Part model, mm, in its own coordinate system. A direction names the side the tool comes from. Give positions to 0.01 mm unless a question says otherwise; leave off trailing zeros. Order: outer loops, then holes, each group sorted by start corner. A loop starts at its lowest first (then second) coordinate and runs counter-clockwise, first axis right, second up. Notation, with made-up numbers: M -22.75,17 L 6.25,17 A36 cw 6.25,52 Z; hole C 52.5,31 d4. An arc over 180 degrees is marked long. Answer as a JSON object with one key per item and string values.
from build123d import *

# Parameters (mm, degrees)
BOSS_EXTRUDE1_DEPTH = 3
FILLET1_R           = 3
SKETCH2_R           = 3
BOSS_EXTRUDE2_DEPTH = 7
SKETCH3_R           = 1.25
CUT_EXTRUDE1_DEPTH  = 11
SKETCH4_R           = 2.125
CUT_EXTRUDE2_DEPTH  = 4


with BuildPart() as part:
    # Sketch1 → Boss-Extrude1 (new body)
    with BuildSketch(Plane(origin=(0, 0, 0), x_dir=(1, 0, 0), z_dir=(0, 1, 0))):
        Polygon((81.303847577, 152.822394855), (113.635462652, 208.822394855), (237.663230149, -6), (173, -6), align=None)
    extrude(amount=BOSS_EXTRUDE1_DEPTH)

    # Fillet1
    fillet1_edges = [part.edges().sort_by_distance(p)[0] for p in [
        (173, 1.5, 6),
        (81.303847577, 1.5, -152.822394855),
        (113.635462652, 1.5, -208.822394855),
        (237.663230149, 1.5, 6),
    ]]
    fillet(fillet1_edges, radius=FILLET1_R)

    # Sketch2 → Boss-Extrude2 (add)
    with BuildSketch(Plane(origin=(0, 3, 0), x_dir=(1, 0, 0), z_dir=(0, 1, 0))):
        with Locations((110.683012702, 108.936188175)):
            Circle(SKETCH2_R)
        with Locations((153.118257487, 133.436188175)):
            Circle(SKETCH2_R)
        with Locations((182.118257487, 83.206714755)):
            Circle(SKETCH2_R)
        with Locations((139.683012702, 58.706714755)):
            Circle(SKETCH2_R)
    extrude(amount=BOSS_EXTRUDE2_DEPTH)

    # Sketch3 → Cut-Extrude1 (cut, through all)
    with BuildSketch(Plane(origin=(0, 10, 0), x_dir=(1, 0, 0), z_dir=(0, 1, 0))):
        with Locations((110.683012702, 108.936188175)):
            Circle(SKETCH3_R)
        with Locations((153.118257487, 133.436188175)):
            Circle(SKETCH3_R)
        with Locations((182.118257487, 83.206714755)):
            Circle(SKETCH3_R)
        with Locations((139.683012702, 58.706714755)):
            Circle(SKETCH3_R)
    extrude(amount=-CUT_EXTRUDE1_DEPTH, mode=Mode.SUBTRACT)

    # Sketch4 → Cut-Extrude2 (cut, through all)
    with BuildSketch(Plane(origin=(0, 3, 0), x_dir=(1, 0, 0), z_dir=(0, 1, 0))):
        with Locations((87.767949192, 152.018547277)):
            Circle(SKETCH4_R)
        with Locations((114.099564267, 197.626242432)):
            Circle(SKETCH4_R)
        with Locations((175.535898385, 0)):
            Circle(SKETCH4_R)
        with Locations((228.199128534, 0)):
            Circle(SKETCH4_R)
    extrude(amount=-CUT_EXTRUDE2_DEPTH, mode=Mode.SUBTRACT)


solid = part.part
1. Which spindle directions (+Z, -Z, +X, -X, +Y, -Y) get a long thin tool onto all of the face, cutting with end or side? Do faces 4 (the flat face through (96.4, 1.48, -178.97)), 5 (the cylindrical face through (154.731, 6.451, -135.966)). Say none if no direction does.
Worked answers:
{"face 4": "-Z, -X, +Y, -Y", "face 5": "+Y"}
2. Pin check, flat tips, straight feed: P1, Ø4, axis at x = 175.54, z = 0, coming from the -Y side; P2, Ø1.5, axis at y = 7, z = -80, coming from the -X side; P3, Ø3, axis at x = 182.12, z = -83.21, coming from the -Y side; P4, Ø4, axis at y = 7.5, z = -135, coming from the +X side. Stop position of each tip, or through.
Worked answers:
{"P1": "passes through", "P2": "stops at x = 180.4", "P3": "stops at y = 0", "P4": "stops at x = 156.12"}
3. Cut at C-C on x = 198.5. Give the cut face in (y, z).
Worked answers:
{"outline": "M 0,-61.83 L 3,-61.83 L 3,6 L 0,6 Z"}
4. Cut at A-A on y = 4.75. Give the cut face in (x, z), plus the area to 3 significant figures.
Worked answers:
{"outline": "C 110.68,-108.94 d6; C 139.68,-58.71 d6; C 153.12,-133.44 d6; C 182.12,-83.21 d6; hole C 110.68,-108.94 d2.5; hole C 139.68,-58.71 d2.5; hole C 153.12,-133.44 d2.5; hole C 182.12,-83.21 d2.5", "area": "93.5 mm^2"}
5. Two-plate mould, pull along X, no slides. Class faces 1 (the cylindrical face through (173.413, 1.521, -0.093)), 2 (the flat face through (153, 10, -132)), 3 (the cylindrical face through (183.503, 6.451, -80.545)): +X half, -X half, draft (parallel to the pull), parting line (faces both ways), or undercut.
Worked answers:
{"face 1": "undercut", "face 2": "draft", "face 3": "parting line"}
6. Cut at B-B on z = -16.5. Give the cut face in (x, y), plus the area to 3 significant figures.
Worked answers:
{"outline": "M 160.01,0 L 224.67,0 L 224.67,3 L 160.01,3 Z", "area": "194 mm^2"}
7. Probe line 1 along X through (y, z) = (1.9, 0); line 2 along Y through (x, z) = (108.5, -154.5); line 3 along X through (y, z) = (1, -81.5). List the from-to ranges inside material, lowest first.
Worked answers:
{"line 1": "x = 169.54 to 173.41, 177.66 to 226.07, 230.32 to 234.2", "line 2": "y = 0 to 3", "line 3": "x = 122.48 to 187.15"}
